Read the model definition and answer for the solid it produces. Units are mm, in the model's axes. A direction names the side the tool comes from. Coordinates: 2 decimals unless noted, no trailing zeros. Write each loop counter-clockwise with the first axis right and the second up, starting at its lowest first coordinate (ties: lowest second). Pieces come first, ordered by that corner, then holes. Notation, with made-up numbers: (82.25, 85.5) -> (117.25, 85.5) arc R22 cw to (117.25, 92.5) -> close; hole circle Ø2 at (-30, 1.25). An arc over 180 degrees is marked (long way). One line per item, written item: value. Start each with the question number.
from build123d import *

# Parameters (mm, degrees)
SKETCH_1_R          = 14
SKETCH_1_R_2        = 4
EXTRUDE_1_DEPTH     = 5
SKETCH_2_R          = 4
SKETCH_2_R_2        = 1.7
EXTRUDE_2_DEPTH     = 7
SKETCH_3_R          = 3.25
CUT_EXTRUDE_1_DEPTH = 4
SKETCH_4_R          = 10
CUT_EXTRUDE_2_DEPTH = 5


with BuildPart() as part:
    # 草图1 → 凸台-拉伸1 (new body)
    with BuildSketch(Plane.XY):
        Circle(SKETCH_1_R)
        Circle(SKETCH_1_R_2, mode=Mode.SUBTRACT)
    extrude(amount=EXTRUDE_1_DEPTH)

    # 草图2 → 凸台-拉伸2 (add)
    with BuildSketch(Plane.XY.offset(5)):
        Polygon((-17.5, 12.905591591), (-12.905591591, 17.5), (12.905591591, 17.5), (17.5, 12.905591591), (17.5, -12.905591591), (12.905591591, -17.5), (-12.905591591, -17.5), (-17.5, -12.905591591), align=None)
        Circle(SKETCH_2_R, mode=Mode.SUBTRACT)
        with Locations((-12.374368671, 12.374368671)):
            Circle(SKETCH_2_R_2, mode=Mode.SUBTRACT)
        with Locations((12.374368671, 12.374368671)):
            Circle(SKETCH_2_R_2, mode=Mode.SUBTRACT)
        with Locations((12.374368671, -12.374368671)):
            Circle(SKETCH_2_R_2, mode=Mode.SUBTRACT)
        with Locations((-12.374368671, -12.374368671)):
            Circle(SKETCH_2_R_2, mode=Mode.SUBTRACT)
    extrude(amount=EXTRUDE_2_DEPTH)

    # 草图3 → 切除-拉伸1 (cut)
    with BuildSketch(Plane.XY.offset(12)):
        with Locations((-12.374368671, 12.374368671)):
            Circle(SKETCH_3_R)
        with Locations((12.374368671, 12.374368671)):
            Circle(SKETCH_3_R)
        with Locations((12.374368671, -12.374368671)):
            Circle(SKETCH_3_R)
        with Locations((-12.374368671, -12.374368671)):
            Circle(SKETCH_3_R)
    extrude(amount=-CUT_EXTRUDE_1_DEPTH, mode=Mode.SUBTRACT)

    # 草图4 → 切除-拉伸2 (cut)
    with BuildSketch(Plane(origin=(0, 0, 0), x_dir=(-1, 0, 0), z_dir=(0, 0, -1))):
        Circle(SKETCH_4_R)
    extrude(amount=-CUT_EXTRUDE_2_DEPTH, mode=Mode.SUBTRACT)


solid = part.part
1. A cutting plane is placed at C-C on z = 9. Give the vertices of the cut face in (x, y).
2. A cutting plane is placed at D-D on y = 13.5. Give the vertices of the cut face in (x, z), then the cut area to 3 significant figures.
3. Find the intervals of material crossed by probe 1 along Y at (x, z) = (-14.5, 8.5); probe 2 along X at (y, z) = (4, 2.5); probe 3 along Y at (x, z) = (-9, 4.25), in increasing order. Write a range as from..to.
4. Given pin 1 (3 mm diameter, centred on x = -12.37, y = 12.37, fed in from -Z); pin 2 (3 mm diameter, centred on x = 12, y = -12.5, fed in from +Z); pin 3 (6 mm diameter, centred on x = 4.5, y = 4.5, fed in from -Z); pin 4 (3 mm diameter, centred on x = 6.5, z = 1.5, fed in from -Y), each flat-ended and moving along its own axis, determine where each tip first touches the part or whether it passes through.
5. For a pull along X with two mould halves and no side action, classify faces 1 (the face through (-15.235, 15.171, 8.451)), 2 (the face through (12.932, -5.362, 2.465)), 3 (the face through (-0.867, -3.905, 8.451)) as +X half, -X half, draft (parallel to the pull), parting line (faces both ways), or undercut.
6. A cutting plane is placed at A-A on y = 0. Give the vertices of the cut face in (x, z), then the cut area to 3 significant figures.
7. A tool of negligible diameter and unlimited length cuts with its end or side. For faces 4 (the face through (0, 17.5, 8)), 5 (the face through (2.17, -9.76, 2.46)), 6 (the face through (14, 11, 8)), from which of +Z, -Z, +X, -X, +Y, -Y can it reach the whole face along a straight path? Write none if from no direction.
Derived:
1. outline: (-17.5, -12.91) -> (-12.91, -17.5) -> (12.91, -17.5) -> (17.5, -12.91) -> (17.5, 12.91) -> (12.91, 17.5) -> (-12.91, 17.5) -> (-17.5, 12.91) -> close; hole circle Ø6.5 at (-12.37, -12.37); hole circle Ø6.5 at (-12.37, 12.37); hole circle Ø8 at (0, 0); hole circle Ø6.5 at (12.37, -12.37); hole circle Ø6.5 at (12.37, 12.37)
2. outline: (-16.91, 5) -> (-13.65, 5) -> (-13.65, 8) -> (-15.42, 8) -> (-15.42, 12) -> (-16.91, 12) -> close; (-11.1, 5) -> (-3.71, 5) -> (-3.71, 0) -> (3.71, 0) -> (3.71, 5) -> (11.1, 5) -> (11.1, 8) -> (9.33, 8) -> (9.33, 12) -> (-9.33, 12) -> (-9.33, 8) -> (-11.1, 8) -> close; (13.65, 5) -> (16.91, 5) -> (16.91, 12) -> (15.42, 12) -> (15.42, 8) -> (13.65, 8) -> close
2. area: 210 mm2
3. probe 1: y = -15.91..-14.83, -9.92..9.92, 14.83..15.91
3. probe 2: x = -13.42..-9.17, 9.17..13.42
3. probe 3: y = -10.72..-4.36, 4.36..10.72
4. pin 1: passes through
4. pin 2: stops at z = 8
4. pin 3: stops at z = 5
4. pin 4: stops at y = -13.08
5. face 1: -X half
5. face 2: parting line
5. face 3: undercut
6. outline: (-17.5, 5) -> (-14, 5) -> (-14, 0) -> (-10, 0) -> (-10, 5) -> (-4, 5) -> (-4, 12) -> (-17.5, 12) -> close; (4, 5) -> (10, 5) -> (10, 0) -> (14, 0) -> (14, 5) -> (17.5, 5) -> (17.5, 12) -> (4, 12) -> close
6. area: 229 mm2
7. face 4: +Z, -Z, +X, -X, +Y
7. face 5: -Z
7. face 6: +Z
